Geometry check sheet. Reference: the model listing, model coordinates, mm. A direction names the side the tool comes from. Round coordinates to 2 decimals unless told otherwise and drop trailing zeros. Write each loop counter-clockwise with the first axis right and the second up, starting at its lowest first coordinate (ties: lowest second). Pieces come first, ordered by that corner, then holes.
Item 1: Cross-section at B-B (z = 7.5). State how many separate pieces and enclosed holes the cut face has, then the cut area to 3 significant figures.
Item 2: Access from +Z, -Z, +X, -X, +Y, -Y to the whole of each face (thin tool, end or side, straight path). Record for faces 1 (the face through (81.02, 32.48, 22.99)), 2 (the face through (54, -117.475, 17)), 3 (the face through (0, -79, -38.989)), 4 (the face through (-17, 71, -9.601)).
Item 3: Scan lines: probe 1 along Z at (x, y) = (40.5, 65); probe 2 along Z at (x, y) = (-5, -41.5); probe 3 along Y at (x, z) = (-16.5, -37.5). Record each from-to range of solid material in increasing order.
Item 4: Draft check along Y on faces 5 (the face through (100.086, -89.102, 17.243)), 6 (the face through (-82.386, 26.067, 11.599)), 7 (the face through (122.96, -54.49, 17.24)), 8 (the face through (11.036, -8.462, -33.951)). Enter one of: pulls with the +Y half, pulls with the -Y half, needs draft (parallel to the pull), parting line crosses it, or undercut.
Item 5: Cross-section at A-A (y = 0). Enter the section's corners in (x, z), then the cut area to 3 significant figures.
Item 6: Depth check by flat-ended pin: P1, Ø1.5, axis at x = 79, y = 27, coming from the +Z side; P2, Ø6, axis at x = 79.89, y = 25.96, coming from the +Z side; P3, Ø6, axis at x = -58, y = -26, coming from the +Z side. Enter the tip coordinate at first touch or a pass-through.
from build123d import *

# Parameters (mm, degrees)
SKETCH1_R                  = 98.2726
EXTRUDE1_DEPTH             = 26.8732
EXTRUDE1_TAPER             = 17.5
SKETCH2_R                  = 2.5
EXTRUDE2_DEPTH             = 22.8854
EXTRUDE3_DEPTH             = 7.874
SKETCH4_W                  = 246.961047875
SKETCH4_H                  = 84.3534
EXTRUDE4_DEPTH             = 7.1374
EXTRUDE4_DIRECTION_2_REACH = 143.553
EXTRUDE5_DEPTH             = 34.0106
EXTRUDE6_DEPTH             = 34.0106
SKETCH8_R                  = 25.7175
EXTRUDE7_DEPTH             = 38.989
SKETCH9_R                  = 79.248
EXTRUDE9_DEPTH             = 9.6012
SKETCH10_R                 = 72.39
EXTRUDE10_DEPTH            = 14.4018
SKETCH11_R                 = 37.592
EXTRUDE11_DEPTH            = 18.9992
SKETCH12_R                 = 13.9065
EXTRUDE12_DEPTH            = 21.717
EXTRUDE13_DEPTH            = 22.4028
CHAMFER1_SIZE              = 5.08
FILLET1_R                  = 10.8331
FILLET2_R                  = 2.54
SKETCH17_R                 = 4.572
EXTRUDE14_DEPTH            = 191.331955682
EXTRUDE15_START            = 3.2639
SKETCH18_R                 = 19.05
SKETCH18_R_2               = 13.9065
EXTRUDE15_DEPTH            = 3.2639


with BuildPart() as part:
    # Sketch1 → Extrude1 (new body)
    with BuildSketch(Plane.XY):
        Circle(SKETCH1_R)
    extrude(amount=EXTRUDE1_DEPTH, taper=EXTRUDE1_TAPER)

    # Sketch2 → Extrude2 (cut)
    with BuildSketch(Plane.XY.offset(26.8732)):
        with Locations((0, 83.9978)):
            Circle(SKETCH2_R)
        with Locations((-79.888747369, 25.957427527)):
            Circle(SKETCH2_R)
        with Locations((79.888747369, 25.957427527)):
            Circle(SKETCH2_R)
    extrude(amount=-EXTRUDE2_DEPTH, mode=Mode.SUBTRACT)

    # Sketch3 → Extrude3 (cut)
    with BuildSketch(Plane.XY.offset(26.8732)):
        with BuildLine():
            Line((-5.8547, 83.9978), (-5.8547, 107.083482694))
            Line((-5.8547, 107.083482694), (5.8547, 107.083482694))
            Line((5.8547, 107.083482694), (5.8547, 83.9978))
            ThreePointArc((5.8547, 83.9978), (0, 78.1431), (-5.8547, 83.9978))
        make_face()
        with BuildLine():
            Line((78.079545572, 31.525578113), (107.519879311, 41.091322409))
            Line((107.519879311, 41.091322409), (110.140650445, 33.912588651))
            Line((110.140650445, 33.912588651), (111.136243984, 29.954358751))
            Line((111.136243984, 29.954358751), (81.697949166, 20.389276942))
            ThreePointArc((81.697949166, 20.389276942), (74.320596783, 24.148225731), (78.079545572, 31.525578113))
        make_face()
        with BuildLine():
            Line((-78.079545572, 31.525578113), (-100.241812355, 38.726535104))
            Line((-100.241812355, 38.726535104), (-103.860215949, 27.590233933))
            Line((-103.860215949, 27.590233933), (-81.697949166, 20.389276942))
            ThreePointArc((-81.697949166, 20.389276942), (-74.320596783, 24.148225731), (-78.079545572, 31.525578113))
        make_face()
    extrude(amount=-EXTRUDE3_DEPTH, mode=Mode.SUBTRACT)

    # Sketch4 → Extrude4 (add)
    with BuildSketch(Plane.XY.offset(26.8732)):
        with Locations((9.213520109, -81.0133)):
            Rectangle(SKETCH4_W, SKETCH4_H)
    extrude(amount=EXTRUDE4_DEPTH)

    # Extrude4 direction 2: up to this face of the body (flat: up to its plane)
    extrude4_direction_2_end = Plane(part.part.faces().sort_by_distance((0, 0, 0))[0])
    # Sketch4 → Extrude4 direction 2 (add, up to the picked face)
    with BuildSketch(Plane.XY.offset(26.8732), mode=Mode.PRIVATE) as extrude4_direction_2_sk1:
        with Locations((9.213520109, -81.0133)):
            Rectangle(SKETCH4_W, SKETCH4_H)
    extrude4_direction_2_tool1 = split(extrude(extrude4_direction_2_sk1.sketch, amount=-EXTRUDE4_DIRECTION_2_REACH, mode=Mode.PRIVATE), bisect_by=extrude4_direction_2_end, keep=Keep.BOTH, mode=Mode.PRIVATE)
    add(extrude4_direction_2_tool1.solids().sort_by(Axis((9.21352, -81.0133, 26.8732), (0, 0, -1)))[0])

    # Sketch5 → Extrude5 (cut)
    with BuildSketch(Plane.XY.offset(34.0106)):
        Polygon((-83.82, -67.2338), (-40.6908, -67.2338), (-40.6908, -176.31524759), (-133.730255454, -176.31524759), (-133.730255454, -141.532127837), (-175.240717896, -141.532127837), (-175.240717896, -38.8366), (-83.82, -38.8366), align=None)
    extrude(amount=-EXTRUDE5_DEPTH, mode=Mode.SUBTRACT)

    # Sketch6 → Extrude6 (cut)
    with BuildSketch(Plane.XY.offset(34.0106)):
        Polygon((40.5892, -117.475), (68.7832, -117.475), (101.0412, -89.6112), (101.0412, -65.5574), (122.9614, -65.5574), (122.9614, -43.8912), (95.504, -43.8912), (95.504, -38.8366), (122.9614, -38.8366), (122.9614, 0), (187.241229942, 0), (187.241229942, -89.6112), (148.373467802, -89.6112), (148.373467802, -112.172308269), (148.373467802, -172.462981515), (68.7832, -172.462981515), (40.5892, -172.462981515), align=None)
    extrude(amount=-EXTRUDE6_DEPTH, mode=Mode.SUBTRACT)

    # Sketch8 → Extrude7 (add)
    with BuildSketch(Plane(origin=(0, 0, 0), x_dir=(-1, 0, 0), z_dir=(0, 0, -1))):
        with Locations(Location((0, -79.0956, 0), (0, 0, 180))):
            Circle(SKETCH8_R)
        with Locations(Location((-47.7266, -57.0992, 0), (0, 0, 180))):
            Circle(SKETCH8_R)
    extrude(amount=EXTRUDE7_DEPTH)

    # Sketch9 → Extrude9 (add)
    with BuildSketch(Plane(origin=(0, 0, 0), x_dir=(-1, 0, 0), z_dir=(0, 0, -1))):
        Circle(SKETCH9_R)
    extrude(amount=EXTRUDE9_DEPTH)

    # Sketch10 → Extrude10 (add)
    with BuildSketch(Plane(origin=(0, 0, -9.6012), x_dir=(-1, 0, 0), z_dir=(0, 0, -1))):
        Circle(SKETCH10_R)
    extrude(amount=EXTRUDE10_DEPTH)

    # Sketch11 → Extrude11 (add)
    with BuildSketch(Plane(origin=(0, 0, -24.003), x_dir=(-1, 0, 0), z_dir=(0, 0, -1))):
        Circle(SKETCH11_R)
    extrude(amount=EXTRUDE11_DEPTH)

    # Sketch12 → Extrude12 (cut)
    with BuildSketch(Plane(origin=(0, 0, -43.0022), x_dir=(-1, 0, 0), z_dir=(0, 0, -1))):
        Circle(SKETCH12_R)
    extrude(amount=-EXTRUDE12_DEPTH, mode=Mode.SUBTRACT)

    # Sketch13 → Extrude13 (add)
    with BuildSketch(Plane(origin=(0, 0, 0), x_dir=(-1, 0, 0), z_dir=(0, 0, -1))):
        with BuildLine():
            Line((-58.491115046, -80.455463016), (-10.764515046, -102.451863016))
            ThreePointArc((-10.764515046, -102.451863016), (23.356263016, -89.860115046), (10.764515046, -55.739336984))
            Line((10.764515046, -55.739336984), (-36.962084954, -33.742936984))
            ThreePointArc((-36.962084954, -33.742936984), (-71.082863016, -46.334684954), (-58.491115046, -80.455463016))
        make_face()
    extrude(amount=EXTRUDE13_DEPTH)

    # Chamfer1
    chamfer1_edges = [part.edges().sort_by_distance(p)[0] for p in [
        (-25.7175, -79.0956, -38.989),
        (22.0091, -57.0992, -38.989),
    ]]
    chamfer(chamfer1_edges, length=CHAMFER1_SIZE)

    # Fillet1
    # the kernel refuses this fillet: 10.8331 mm, written as the material it adds along each edge
    with BuildSketch(Plane(origin=(101.0412, -65.5574, 34.0106), x_dir=(1, 0, 0), z_dir=(0, 0, -1)), Plane(origin=(-40.6908, -67.2338, 34.0106), x_dir=(0, -1, 0), z_dir=(0, 0, -1))) as fillet1_piece_1:
        with BuildLine():
            CenterArc((FILLET1_R, FILLET1_R), FILLET1_R, 180, 90)
            Line((0, FILLET1_R), (0, 0))
            Line((0, 0), (FILLET1_R, 0))
        make_face()
    extrude(amount=34.0106)
    # the kernel refuses this fillet: 10.8331 mm, written as the material it takes off along each edge
    with BuildSketch(Plane(origin=(122.9614, -65.5574, 61.09335), x_dir=(0, 1, 0), z_dir=(0, 0, -1)), Plane(origin=(122.9614, -43.8912, 61.09335), x_dir=(-1, 0, 0), z_dir=(0, 0, -1)), Plane(origin=(-83.82, -67.2338, 61.09335), x_dir=(1, 0, 0), z_dir=(0, 0, -1))) as fillet1_2_piece_1:
        with BuildLine():
            CenterArc((FILLET1_R, -FILLET1_R), FILLET1_R, 90, 90)
            Line((0, -FILLET1_R), (0, 0))
            Line((0, 0), (FILLET1_R, 0))
        make_face()
    extrude(amount=88.1761, mode=Mode.SUBTRACT)
    with BuildSketch(Plane(origin=(101.0412, -89.6112, 46.404396211), x_dir=(0, 1, 0), z_dir=(0, 0, -1))) as fillet1_2_piece_2:
        with BuildLine():
            CenterArc((FILLET1_R * 0.457626947463, -FILLET1_R), FILLET1_R, 90, 49.180218113)
            Line((-FILLET1_R * 0.299142463693, -FILLET1_R * 0.346318075561), (0, 0))
            Line((0, 0), (FILLET1_R * 0.457626947463, 0))
        make_face()
    extrude(amount=58.798192423, mode=Mode.SUBTRACT)
    with BuildSketch(Plane(origin=(68.7832, -117.475, 44.08790669), x_dir=(0.7567694111558876, 0.6536819244393799, 0), z_dir=(0, 0, -1))) as fillet1_2_piece_3:
        with BuildLine():
            CenterArc((FILLET1_R * 0.372093184392, -FILLET1_R), FILLET1_R, 90, 40.819781887)
            Line((-FILLET1_R * 0.281588740047, -FILLET1_R * 0.243230588844), (0, 0))
            Line((0, 0), (FILLET1_R * 0.372093184392, 0))
        make_face()
    extrude(amount=54.165213379, mode=Mode.SUBTRACT)
    with BuildSketch(Plane(origin=(-40.6908, -123.19, -27.08275), x_dir=(1, 0, 0), z_dir=(0, 0, 1))) as fillet1_2_piece_4:
        with BuildLine():
            CenterArc((FILLET1_R, FILLET1_R), FILLET1_R, 180, 90)
            Line((0, FILLET1_R), (0, 0))
            Line((0, 0), (FILLET1_R, 0))
        make_face()
    extrude(amount=88.1761, mode=Mode.SUBTRACT)

    # Fillet2
    fillet2_edges = [part.edges().sort_by_distance(p)[0] for p in [
        (40.5892, -123.19, 17.0053),
        (40.5892, -117.475, 17.0053),
    ]]
    fillet(fillet2_edges, radius=FILLET2_R)

    # Sketch17 → Extrude14 (cut, through all)
    with BuildSketch(Plane.XY.offset(34.0106)):
        with Locations((-72.9996, -55.2958)):
            Circle(SKETCH17_R)
        with Locations((112.000400002, -55.2958)):
            Circle(SKETCH17_R)
        with Locations((-29.999599996, -112.295800021)):
            Circle(SKETCH17_R)
    extrude(amount=-EXTRUDE14_DEPTH, mode=Mode.SUBTRACT)

    # Sketch18 → Extrude15 (add)
    with BuildSketch(Plane(origin=(0, 0, -43.0022), x_dir=(-1, 0, 0), z_dir=(0, 0, -1)).offset(EXTRUDE15_START)):
        with Locations(Location((0, 0, 0), (0, 0, 180))):
            Circle(SKETCH18_R)
        Circle(SKETCH18_R_2, mode=Mode.SUBTRACT)
    extrude(amount=-EXTRUDE15_DEPTH)


solid = part.part
Resolved:
1. separate pieces: 1
1. enclosed holes: 6
1. area: 34,200 mm2
2. face 1: +Z, +X
2. face 2: +Z, -Z, +X, -Y
2. face 3: -Z, +X, -X, -Y
2. face 4: -Z
3. probe 1: z = -9.6 to 26.87
3. probe 2: z = -24 to 34.01
3. probe 3: y = -93.84 to -64.35, -33.78 to 33.78
4. face 5: pulls with the -Y half
4. face 6: undercut
4. face 7: parting line crosses it
4. face 8: undercut
5. outline: (-98.27, 0) - (-79.25, 0) - (-79.25, -9.6) - (-72.39, -9.6) - (-72.39, -24) - (-37.59, -24) - (-37.59, -43) - (-19.05, -43) - (-19.05, -46.27) - (-13.91, -46.27) - (-13.91, -21.29) - (13.91, -21.29) - (13.91, -46.27) - (19.05, -46.27) - (19.05, -43) - (37.59, -43) - (37.59, -24) - (72.39, -24) - (72.39, -9.6) - (79.25, -9.6) - (79.25, 0) - (98.27, 0) - (89.8, 26.87) - (-89.8, 26.87) - close
5. area: 9,520 mm2
6. P1: stops at z = 3.99
6. P2: stops at z = 19
6. P3: stops at z = 26.87
